The model under review builds one solid part; all positions refer to its coordinate system, in mm. A direction names the side the tool comes from. Coordinates: 2 decimals unless noted, no trailing zeros. Write each loop counter-clockwise with the first axis right and the second up, starting at its lowest first coordinate (ties: lowest second). Pieces come first, ordered by that corner, then holes. Notation, with made-up numbers: (86, -10) -> (118, -10) arc R27 cw to (118, 17) -> close; hole circle Ø6 at (3.25, -12). An arc over 180 degrees is marked (long way). Put each result on its own line as item: value. Start each with the question number.
from build123d import *

# Parameters (mm, degrees)
BASE_FLANGE1_START      = -1
BASE_FLANGE1_OUTLINE_W  = 100
BASE_FLANGE1_OUTLINE_H  = 30
BASE_FLANGE1_DEPTH      = 2
EDGE_FLANGE1_DEPTH      = 30
EDGE_FLANGE1_START      = 2
EDGE_FLANGE1_FLAT_DEPTH = 2
SKETCH11_R              = 6
CUT_EXTRUDE2_DEPTH      = 2
EDGE_FLANGE2_DEPTH      = 35.375352101
CUT_EXTRUDE1_DEPTH      = 10
CHAMFER1_SIZE           = 8


# Read off the part's stored shape, not the designer's step: Base-Flange1
# Sheet-metal steps are written as plain solids
with BuildPart() as part:
    # Base-Flange1 outline → Base-Flange1 (new body)
    with BuildSketch(Plane(origin=(0, 0, 0), x_dir=(0, 1, 0), z_dir=(0, 0, 1)).offset(BASE_FLANGE1_START)):
        with Locations((50, 15)):
            Rectangle(BASE_FLANGE1_OUTLINE_W, BASE_FLANGE1_OUTLINE_H)
    extrude(amount=BASE_FLANGE1_DEPTH)

    # Edge-Flange1 bend section (across the edge) → Edge-Flange1 (add)
    with BuildSketch(Plane(origin=(2, 70, 1), x_dir=(-1, 0, 0), z_dir=(0, 1, 0))):
        with BuildLine():
            Line((-2, 2), (0, 2))
            ThreePointArc((0, 2), (0.585786438, 0.585786438), (2, 0))
            Line((2, 0), (2, -2))
            ThreePointArc((2, -2), (-0.828427125, -0.828427125), (-2, 2))
        make_face()
    extrude(amount=EDGE_FLANGE1_DEPTH)

    # Edge-Flange1 profile (on flange) → Edge-Flange1 flat (add)
    with BuildSketch(Plane(origin=(2, 0, 1), x_dir=(0, 1, 0), z_dir=(1, 0, 0)).offset(EDGE_FLANGE1_START)):
        Polygon((70, 2), (100, 2), (100, 43), (70, 24.253919443), align=None)
    extrude(amount=-EDGE_FLANGE1_FLAT_DEPTH)

    # Sketch11 → Cut-Extrude2 (cut)
    with BuildSketch(Plane.XY.offset(1)):
        with Locations((-15, 16)):
            Circle(SKETCH11_R)
    extrude(amount=-CUT_EXTRUDE2_DEPTH, mode=Mode.SUBTRACT)

    # Edge-Flange2 section (across the edge) → Edge-Flange2 (add)
    with BuildSketch(Plane(origin=(4, 98.940161472, 45.696096192), x_dir=(0, 0.5299192642332061, -0.8480480961564253), z_dir=(-1.8389111764499846e-15, -0.8480480961564253, -0.5299192642332061))):
        with BuildLine():
            Line((-2, 2), (-2, 36))
            Line((-2, 36), (0, 36))
            Line((0, 36), (0, 2))
            ThreePointArc((0, 2), (0.585786438, 0.585786438), (2, 0))
            Line((2, 0), (2, -2))
            ThreePointArc((2, -2), (-0.828427125, -0.828427125), (-2, 2))
        make_face()
    extrude(amount=EDGE_FLANGE2_DEPTH)

    # Sketch15 → Cut-Extrude1 (cut)
    with BuildSketch(Plane(origin=(0, 6.188296585, -9.903344701), x_dir=(1, 0, 0), z_dir=(0, -0.5299192642332063, 0.8480480961564252))):
        with BuildLine():
            Line((31, 92.745905141), (31, 86.745905141))
            ThreePointArc((31, 86.745905141), (25, 80.745905141), (19, 86.745905141))
            Line((19, 86.745905141), (19, 92.745905141))
            ThreePointArc((19, 92.745905141), (25, 98.745905141), (31, 92.745905141))
        make_face()
    extrude(amount=-CUT_EXTRUDE1_DEPTH, mode=Mode.SUBTRACT)

    # Chamfer1
    chamfer1_edges = [part.edges().sort_by_distance(p)[0] for p in [
        (40, 98.410242207, 46.544144288),
        (40, 68.410242207, 27.798063731),
    ]]
    chamfer(chamfer1_edges, length=CHAMFER1_SIZE)

    # SurfaceCut1
    split(bisect_by=Plane.YZ.offset(-15), keep=Keep.TOP)

    # Mirror1: part across plane


with BuildPart() as part_1:
    add(part.part)
    add(part.part.mirror(Plane(origin=(-15, 0, 0), x_dir=(0, 0, 1), z_dir=(1, 0, 0))))


solid = part_1.part
1. The part is to be moulded in two halves that separate along X. For faces 6 (the flat face through (4, 85, 19)), 7 (the flat face through (-61, 83, 37)), 8 (the cylindrical face through (-33.14, 83.73, 37.13)), 9 (the cylindrical face through (-32.797, 84.79, 0.141)), say which applies: released by +X, released by -X, zero draft, split by the parting line, or undercut.
2. Wall thickness on line 1 (Y direction, x = -15, z = 0); line 2 (X direction, y = 16, z = 0); line 3 (X direction, y = 81, z = 20.5): over which ranges is each line inside the solid? List them lowest first. Write a range as from..to.
3. Insertion check: P1, Ø6, axis at x = -52, z = 25.5, coming from the -Y side; P2, Ø15, axis at y = 88.5, z = 23.5, coming from the +X side; P3, Ø1.6, axis at y = 44, z = -0.5, coming from the -X side; P4, Ø7, axis at x = -15, y = 16, coming from the +Z side. Each pin has a flat end and moves straight along its axis. Give the tip position at first contact, or say it passes through.
4. Consider section C-C on y = 39.5. State the section outline as (x, z) points, then the cut area to 3 significant figures.
5. Tool access review of faces 1 (the flat face through (15.682, 84.15, 36.454)), 2 (the flat face through (17.2, 98.5, 46.4)), 3 (the flat face through (-34, 85, 19)), 4 (the cylindrical face through (3.14, 83.73, 37.13)), 5 (the flat face through (2, 85, 19)): name each direction out of +Z, -Z, +X, -X, +Y, -Y from which nothing blocks a thin tool from reaching the whole face with its end or side.
6. Consider section B-B on y = 16. State the section outline as (x, z) points.
7. Consider section A-A on x = -15. State the section outline as (y, z) points.
Output values:
1. face 6: released by +X
1. face 7: undercut
1. face 8: undercut
1. face 9: released by -X
2. line 1: y = 0..10, 22..100
2. line 2: x = -30..-21, -9..0
2. line 3: x = -34..-32, 2..4
3. P1: stops at y = 67.97
3. P2: stops at x = 4
3. P3: stops at x = -30
3. P4: passes through
4. outline: (-30, -1) -> (0, -1) -> (0, 1) -> (-30, 1) -> close
4. area: 60.0 mm^2
5. face 1: -Z, +X, +Y
5. face 2: +Z, +X, -X, +Y
5. face 3: -Z, -X, +Y
5. face 4: +Z, -Y
5. face 5: +Z, +Y, -Y
6. outline: (-30, -1) -> (-21, -1) -> (-21, 1) -> (-30, 1) -> close; (-9, -1) -> (0, -1) -> (0, 1) -> (-9, 1) -> close
7. outline: (0, -1) -> (10, -1) -> (10, 1) -> (0, 1) -> close; (22, -1) -> (100, -1) -> (100, 1) -> (22, 1) -> close
